```python
from build123d import *

# Parameters (mm, degrees)
SKETCH_3_W              = 7
SKETCH_3_H              = 12
CONTINUOUS_TONGUE_DEPTH = 5
SKETCH_4_W              = 7
SKETCH_4_H              = 12
EXTRUDE_2_DEPTH         = 5


with BuildPart() as part:
    # 草图1 → Round_nut (revolve)
    with BuildSketch(Plane.XY, mode=Mode.PRIVATE) as round_nut_sk:
        Polygon((4.2, 0), (9, 0), (9, 1), (10, 1), (10, 15), (9, 15), (9, 16), (4.2, 16), align=None)
    revolve(round_nut_sk.sketch.rotate(Axis((0, 0, 0), (0, 1, 0)), 90), axis=Axis((0, 0, 0), (0, 1, 0)))

    # 草图3 → Continuous_tongue (add)
    with BuildSketch(Plane.XY.offset(-2.5)):
        with Locations((-11.5, 8)):
            Rectangle(SKETCH_3_W, SKETCH_3_H)
    extrude(amount=CONTINUOUS_TONGUE_DEPTH)

    # 草图4 → 凸台-拉伸2 (add)
    with BuildSketch(Plane.XY.offset(-2.5)):
        with Locations((11.5, 8)):
            Rectangle(SKETCH_4_W, SKETCH_4_H)
    extrude(amount=EXTRUDE_2_DEPTH)


solid = part.part
```
Read the model definition and answer for the solid it produces. Units are mm, in the model's axes. A direction names the side the tool comes from. Give positions to 0.01 mm unless a question says otherwise; leave off trailing zeros. Write each loop counter-clockwise with the first axis right and the second up, starting at its lowest first coordinate (ties: lowest second). Pieces come first, ordered by that corner, then holes. Notation, with made-up numbers: M 83,48.25 L 113,48.25 A26 ccw 113,66.25 Z; hole C -17,69.25 d4. An arc over 180 degrees is marked long. Put each result on its own line as item: value. Start each with the question number.
1. The part is cut by section B-B, the plane y = 9. Give the vertices of the cut face in (x, z), and give its area (3 significant figures).
2. For a pull along Z with two mould halves and no side action, classify faces 1 (the flat face through (12, 8, 2.5)), 2 (the cylindrical face through (-1.262, 7.888, -4.006)), 3 (the cylindrical face through (-6.083, 15.507, 6.633)), 4 (the flat face through (-2, 1, -9)) as released by +Z, released by -Z, zero draft, split by the parting line, or undercut.
3. Which of the six approach directions +Z, -Z, +X, -X, +Y, -Y give full straight-line access (tool end or side, diameter ignored) to faces 5 (the flat face through (-12, 8, -2.5)), 6 (the cylindrical face through (-6.083, 0.507, 6.633)), 7 (the flat face through (-2, 15, 9)), 8 (the flat face through (-12, 8, 2.5))?
4. Each of these flat-tipped pins is pushed along its axis until it touches: pin 1 Ø2.5 at (x, y) = (-12.5, 5.5) entering from -Z; pin 2 Ø5 at (x, y) = (6.5, 4.5) entering from +Z; pin 3 Ø4 at (x, y) = (-7.5, 2) entering from +Z; pin 4 Ø10 at (x, z) = (4.5, 4) entering from -Y. Where does it stop, or does it pass through?
5. The part is cut by section A-A, the plane x = 0. Give the vertices of the cut face in (y, z), and give its area (3 significant figures).
6. The part is cut by section C-C, the plane z = 0. Give the vertices of the cut face in (x, y).
7. Consider line 1 along X through (y, z) = (9.5, 0); line 2 along Y through (x, z) = (9.75, 1); line 3 along Z through (x, y) = (-0.75, 11). Determine where each line is inside the solid, lowest interval first.
8. The part is cut by section D-D, the plane z = -7.25. Give the vertices of the cut face in (x, y), and give its area (3 significant figures).
Final values:
1. outline: M -15,-2.5 L -9.68,-2.5 A10 ccw 9.68,-2.5 L 15,-2.5 L 15,2.5 L 9.68,2.5 A10 ccw -9.68,2.5 L -15,2.5 Z; hole C 0,0 d8.4
1. area: 310 mm²
2. face 1: released by +Z
2. face 2: undercut
2. face 3: split by the parting line
2. face 4: zero draft
3. face 5: -Z, -X, +Y, -Y
3. face 6: -Y
3. face 7: +Y
3. face 8: +Z, -X, +Y, -Y
4. pin 1: stops at z = -2.5
4. pin 2: stops at z = 9.17
4. pin 3: stops at z = 8.35
4. pin 4: stops at y = 0
5. outline: M 0,-9 L 1,-9 L 1,-10 L 15,-10 L 15,-9 L 16,-9 L 16,-4.2 L 0,-4.2 Z; M 0,4.2 L 16,4.2 L 16,9 L 15,9 L 15,10 L 1,10 L 1,9 L 0,9 Z
5. area: 182 mm²
6. outline: M -15,2 L -10,2 L -10,1 L -9,1 L -9,0 L -4.2,0 L -4.2,16 L -9,16 L -9,15 L -10,15 L -10,14 L -15,14 Z; M 4.2,0 L 9,0 L 9,1 L 10,1 L 10,2 L 15,2 L 15,14 L 10,14 L 10,15 L 9,15 L 9,16 L 4.2,16 Z
7. line 1: x = -15 to -4.2, 4.2 to 15
7. line 2: y = 1 to 15
7. line 3: z = -9.97 to -4.13, 4.13 to 9.97
8. outline: M -6.89,1 L -5.33,1 L -5.33,0 L 5.33,0 L 5.33,1 L 6.89,1 L 6.89,15 L 5.33,15 L 5.33,16 L -5.33,16 L -5.33,15 L -6.89,15 Z
8. area: 214 mm²
